CAD build for the part. Positions are in the model's coordinates, mm. A direction names the side the tool comes from. Coordinates: 2 decimals unless noted, no trailing zeros. Write each loop counter-clockwise with the first axis right and the second up, starting at its lowest first coordinate (ties: lowest second). Pieces come first, ordered by that corner, then holes. Notation, with made-up numbers: (56.5, -16.75) -> (99.5, -16.75) arc R31 ccw to (99.5, 10.25) -> close; hole circle Ø8 at (89.25, 86.5). An arc over 180 degrees is marked (long way). Answer as CSV lines item,"result".
Autodesk Inventor part; units mm, degrees
ref_plane "YZ Plane" through (0, 0, 0) normal (1, 0, 0) x (0, 1, 0)
ref_plane "XZ Plane" through (0, 0, 0) normal (0, 1, 0) x (-1, 0, 0)
ref_plane "XY Plane" through (0, 0, 0) normal (0, 0, 1) x (1, 0, 0)
sketch "Sketch2" plane through (0, 0, 0) normal (1, 0, 0) x (0, 1, 0)
  circle A0 centre (0, 0) radius 7
  circle A1 centre (0, 0) radius 6
  dimension "d0" = 14
  dimension "d1" = 12
extrude "Extrusion1" add sketch "Sketch2" along normal blind 35 contours A1
extrude "Extrusion2" add sketch "Sketch2" along normal blind 7 contours A0 | A1
fillet "Fillet1" radius 1 1 edges at (35, -6, 0)
thread "Thread1"
properties part number "bolt" material "Steel, Cast"
Item 1: Saw through at C-C on x = 3.5. Give the cut face in (y, z), and give its area (3 significant figures).
Answer below:
outline,"circle Ø14 at (0, 0)"
area,"154 mm2"
Item 2: Flat gauge pins, fed straight in: pin 1 (5 mm diameter, centred on x = 3.5, y = -5, fed in from +Z); pin 2 (3 mm diameter, centred on y = 4.5, z = -1, fed in from -X); pin 3 (1.5 mm diameter, centred on x = 16.5, z = 0, fed in from +Y); pin 4 (2 mm diameter, centred on x = 12.5, z = 5.5, fed in from +Y). Where does each tip first touch, or does it go through?
Answer below:
pin 1,"stops at z = 6.54"
pin 2,"stops at x = 0"
pin 3,"stops at y = 6"
pin 4,"stops at y = 3.97"
Item 3: 3-axis set-ups, long thin cutter, end or side, ignore diameter. For faces 1 (the flat face through (7, 6, 2)), 2 (the cylindrical face through (3.451, 6.466, 2.681)): which of +Z, -Z, +X, -X, +Y, -Y reach the whole face in a straight line?
Answer below:
face 1,"+X"
face 2,"+X, -X"
Item 4: Wall check: line 1 (Z direction, x = 13.5, y = 0.25); line 2 (X direction, y = 5, z = -4.75). Give the ranges that are in metal, low to high. Write a range as from..to.
Answer below:
line 1,"z = -5.99..5.99"
line 2,"x = 0..7"
Item 5: Saw through at D-D on x = 30. Give the cut face in (y, z).
Answer below:
outline,"circle Ø12 at (0, 0)"
Item 6: Saw through at A-A on z = 0. Give the cut face in (x, y).
Answer below:
outline,"(0, -7) -> (7, -7) -> (7, -6) -> (34, -6) arc R1 ccw to (35, -5) -> (35, 5) arc R1 ccw to (34, 6) -> (7, 6) -> (7, 7) -> (0, 7) -> close"
